Part model, mm, in its own coordinate system. Coordinates: 2 decimals unless noted, no trailing zeros. Order: outer loops, then holes, each group sorted by start corner. A loop starts at its lowest first (then second) coordinate and runs counter-clockwise, first axis right, second up.
1) Cut at C-C (z = -2.5). List the corners of the cut face in (x, y).
2) Cut at B-B (y = 5.25). List the corners of the cut face in (x, z).
3) Cut at A-A (z = -11). List the corners of the cut face in (x, y), and give its area (3 significant figures).
4) Wall check: L1, parallel to X at y = 3.75, z = 15.5. Give the ranges that are in metal, low to high.
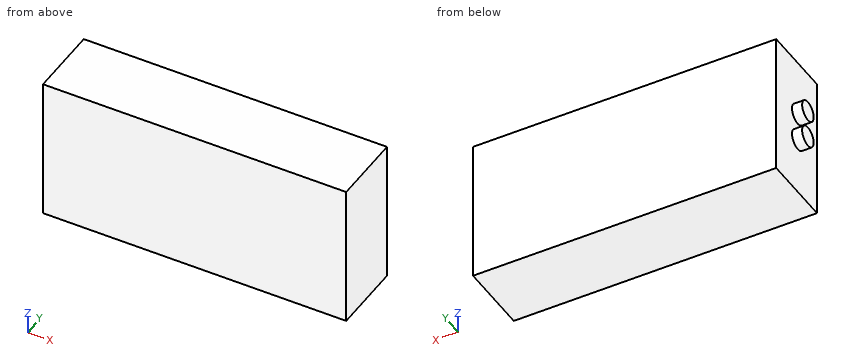
```python
from build123d import *

# Parameters (mm, degrees)
SKETCH1_W           = 75.946
SKETCH1_H           = 36.068
BOSS_EXTRUDE1_DEPTH = 18.034
SKETCH2_R           = 2.54
BOSS_EXTRUDE2_DEPTH = 2.54


with BuildPart() as part:
    # Sketch1 → Boss-Extrude1 (new body)
    with BuildSketch(Plane(origin=(0, 0, 0), x_dir=(1, 0, 0), z_dir=(0, 1, 0))):
        Rectangle(SKETCH1_W, SKETCH1_H)
    extrude(amount=BOSS_EXTRUDE1_DEPTH)

    # Sketch2 → Boss-Extrude2 (add)
    with BuildSketch(Plane.ZY.offset(37.973)):
        with Locations((-3.556, 8.509)):
            Circle(SKETCH2_R)
        with Locations(Location((3.556, 8.509, 0), (0, 0, 180))):
            Circle(SKETCH2_R)
    extrude(amount=BOSS_EXTRUDE2_DEPTH)


solid = part.part
```
Geometry check:
1. outline: (-40.51, 6.2) - (-37.97, 6.2) - (-37.97, 0) - (37.97, 0) - (37.97, 18.03) - (-37.97, 18.03) - (-37.97, 10.82) - (-40.51, 10.82) - close
2. outline: (-37.97, -18.03) - (37.97, -18.03) - (37.97, 18.03) - (-37.97, 18.03) - close
3. outline: (-37.97, 0) - (37.97, 0) - (37.97, 18.03) - (-37.97, 18.03) - close
3. area: 1,370 mm2
4. L1: x = -37.97 to 37.97
